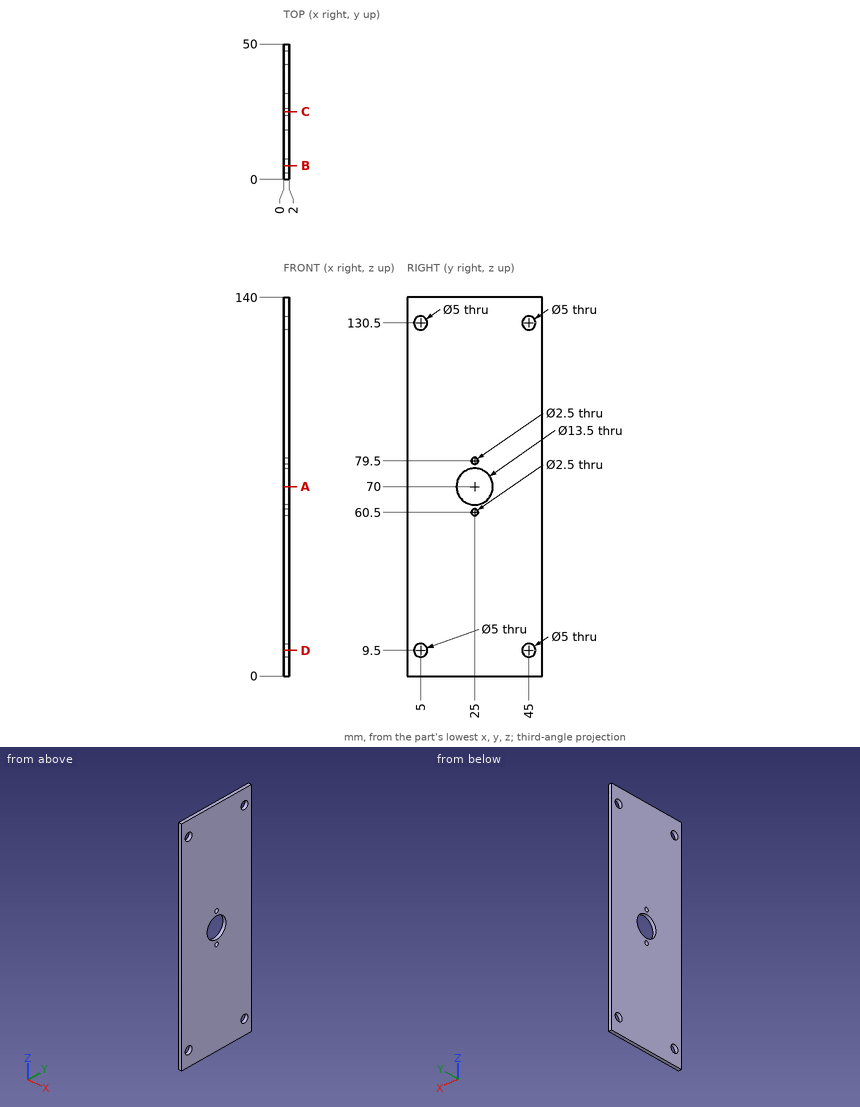
Answer from the drawing. Dimensions are ordinates in mm from the lowest x, y and z of the part. Coordinates: 2 decimals unless noted, no trailing zeros. Write each loop counter-clockwise with the first axis right and the second up, starting at its lowest first coordinate (ties: lowest second). Pieces come first, ordered by that corner, then holes. Notation, with made-up numbers: (46, -25.5) -> (83, -25.5) arc R27 ccw to (83, -9.5) -> close; hole circle Ø8 at (-31, 1.25). An arc over 180 degrees is marked (long way). One line per question, with ' | ' between items.
1. Section A-A (z = 70) is taken. Determine the outline of the cut face in (x, y), and give its area (3 significant figures).
Verdict:
outline: (0, 0) -> (2, 0) -> (2, 18.25) -> (0, 18.25) -> close; (0, 31.75) -> (2, 31.75) -> (2, 50) -> (0, 50) -> close | area: 73.0 mm^2
2. Section C-C (y = 25) is taken. Determine the outline of the cut face in (x, z).
Verdict:
outline: (0, 0) -> (2, 0) -> (2, 59.25) -> (0, 59.25) -> close; (0, 61.75) -> (2, 61.75) -> (2, 63.25) -> (0, 63.25) -> close; (0, 76.75) -> (2, 76.75) -> (2, 78.25) -> (0, 78.25) -> close; (0, 80.75) -> (2, 80.75) -> (2, 140) -> (0, 140) -> close
3. Given pin 1 Ø2 at (y, z) = (25, 79.5) entering from +X, flat-ended and moving along its own axis, determine where the tip first touches the part or whether it passes through.
Verdict:
pin 1: passes through
4. Section D-D (z = 9.5) is taken. Determine the outline of the cut face in (x, y).
Verdict:
outline: (0, 0) -> (2, 0) -> (2, 2.5) -> (0, 2.5) -> close; (0, 7.5) -> (2, 7.5) -> (2, 42.5) -> (0, 42.5) -> close; (0, 47.5) -> (2, 47.5) -> (2, 50) -> (0, 50) -> close
5. Section B-B (y = 5) is taken. Determine the outline of the cut face in (x, z), and give its area (3 significant figures).
Verdict:
outline: (0, 0) -> (2, 0) -> (2, 7) -> (0, 7) -> close; (0, 12) -> (2, 12) -> (2, 128) -> (0, 128) -> close; (0, 133) -> (2, 133) -> (2, 140) -> (0, 140) -> close | area: 260 mm^2
6. Straight lines are drawn through the part: line 1 (Y direction, x = 0.65, z = 130.5); line 2 (Z direction, x = 1.65, y = 46); line 3 (Y direction, x = 0.75, z = 60.5). For each, find the intervals that lie inside material, in ascending order.
Verdict:
line 1: y = 0 to 2.5, 7.5 to 42.5, 47.5 to 50 | line 2: z = 0 to 7.21, 11.79 to 128.21, 132.79 to 140 | line 3: y = 0 to 23.75, 26.25 to 50
